from build123d import *

# Parameters (mm, degrees)
SKETCH_1_W               = 100
SKETCH_1_H               = 10
EXTRUDE_1_DEPTH          = 30
CUT_EXTRUDE_1_DEPTH      = 105.880884817
CUT_EXTRUDE_1_DEPTH_BACK = 105.880884817
SKETCH_2_R               = 2.05
SKETCH_4_W               = 70.552340153
SKETCH_4_H               = 8.779398974
EXTRUDE_2_DEPTH          = 22.5


with BuildPart() as part:
    # 스케치1 → 보스-돌출1 (new, symmetric)
    with BuildSketch(Plane(origin=(0, 0, 0), x_dir=(0, 0, -1), z_dir=(1, 0, 0))):
        with Locations((50, 5)):
            Rectangle(SKETCH_1_W, SKETCH_1_H)
    extrude(amount=EXTRUDE_1_DEPTH, both=True)

    # 스케치2 → 컷-돌출1 (cut, two sides: drawn at the far end of the back side and taken through both)
    with BuildSketch(Plane(origin=(0, 0, 0), x_dir=(0, 0, -1), z_dir=(1, 0, 0)).offset(-CUT_EXTRUDE_1_DEPTH_BACK)):
        with Locations((41.137955169, 5)):
            Circle(SKETCH_2_R)
        with Locations((91.137955169, 5)):
            Circle(SKETCH_2_R)
    extrude(amount=CUT_EXTRUDE_1_DEPTH + CUT_EXTRUDE_1_DEPTH_BACK, mode=Mode.SUBTRACT)

    # 스케치4 → 보스-돌출2 (add, symmetric)
    with BuildSketch(Plane(origin=(0, 0, 0), x_dir=(0, 0, -1), z_dir=(1, 0, 0))):
        with Locations((35.576558904, 14.389699487)):
            Rectangle(SKETCH_4_W, SKETCH_4_H)
    extrude(amount=EXTRUDE_2_DEPTH, both=True)


solid = part.part
Geometry: final body of the model. Coordinates: model frame, mm. A direction names the side the tool comes from. Round coordinates to 2 decimals unless told otherwise and drop trailing zeros. Loops run counter-clockwise (first coordinate to the right, second up) from the corner with the lowest first, then second, coordinate; pieces in that order, holes last.
Q1. Section D-D on y = 13.25. Return loops of the section in (x, z), plus the area to 3 significant figures.
Q2. Material intervals for L1, parallel to Z at x = 9, y = 5; L2, parallel to Z at x = -0.5, y = 6; L3, parallel to X at y = 16.5, z = -11.5, sorted ascending.
Q3. Pull-direction query (Z, two-part tool) for faces 6 (the flat face through (0, 5, -100)), 7 (the cylindrical face through (-0.4, 5.6, -43.1)), 8 (the flat face through (-30, 5, -49)), 9 (the cylindrical face through (-0.42, 5.09, -89.09)); classes: released by +Z, released by -Z, zero draft, split by the parting line, or undercut.
Q4. Section B-B on x = -14. Return loops of the section in (y, z).
Q5. Section C-C on z = -18.5. Return loops of the section in (x, y), plus the area to 3 significant figures.
Q6. Section A-A on y = 5. Return loops of the section in (x, z).
Q7. Access query for faces 1 (the flat face through (30, 5, -49)), 2 (the flat face through (0, 14, -70.853)), 3 (the flat face through (22.5, 14, -35)), 4 (the flat face through (-22.5, 14, -35)), 5 (the flat face through (0, 14, -0.3)). Directions: +Z, -Z, +X, -X, +Y, -Y. A direction counts if a zero-diameter tool reaches every point of the face in a straight line with its end or side. Return the directions, or none.
Q8. Pin query (flat end, axial travel): P1, Ø9.5, axis at y = 15, z = -40, coming from the +X side; P2, Ø2, axis at x = -16.5, z = -12.5, coming from the -Y side; P3, Ø2.5, axis at y = 13.5, z = -44.5, coming from the -X side; P4, Ø2.5, axis at x = -9.5, y = 12.5, coming from the +Z side. Return the tip coordinate at first contact, or that it passes through.
Evaluation:
1. outline: (-22.5, -70.85) - (22.5, -70.85) - (22.5, -0.3) - (-22.5, -0.3) - close
1. area: 3,170 mm2
2. L1: z = -100 to -93.19, -89.09 to -43.19, -39.09 to 0
2. L2: z = -100 to -92.93, -89.35 to -42.93, -39.35 to 0
2. L3: x = -22.5 to 22.5
3. face 6: released by -Z
3. face 7: undercut
3. face 8: zero draft
3. face 9: undercut
4. outline: (0, -100) - (10, -100) - (10, -70.85) - (18.78, -70.85) - (18.78, -0.3) - (10, -0.3) - (10, 0) - (0, 0) - close; hole circle Ø4.1 at (5, -91.14); hole circle Ø4.1 at (5, -41.14)
5. outline: (-30, 0) - (30, 0) - (30, 10) - (22.5, 10) - (22.5, 18.78) - (-22.5, 18.78) - (-22.5, 10) - (-30, 10) - close
5. area: 995 mm2
6. outline: (-30, -100) - (30, -100) - (30, -93.19) - (-30, -93.19) - close; (-30, -89.09) - (30, -89.09) - (30, -43.19) - (-30, -43.19) - close; (-30, -39.09) - (30, -39.09) - (30, 0) - (-30, 0) - close
7. face 1: +Z, -Z, +X, +Y, -Y
7. face 2: -Z, +X, -X, +Y
7. face 3: +Z, -Z, +X, +Y
7. face 4: +Z, -Z, -X, +Y
7. face 5: +Z, +X, -X, +Y
8. P1: stops at x = 22.5
8. P2: stops at y = 0
8. P3: stops at x = -22.5
8. P4: stops at z = -0.3
